Autodesk Inventor part; units mm, degrees
ref_plane "YZ Plane" through (0, 0, 0) normal (1, 0, 0) x (0, 1, 0)
ref_plane "XZ Plane" through (0, 0, 0) normal (0, 1, 0) x (-1, 0, 0)
ref_plane "XY Plane" through (0, 0, 0) normal (0, 0, 1) x (1, 0, 0)
sketch "Sketch2" plane through (0, 0, 0) normal (1, 0, 0) x (0, 1, 0)
  line L0 (0, 0) -> (1, 0)
  line L1 (1, 0) -> (1, 1)
  line L2 (1, 1) -> (2.25, 1)
  line L3 (2.25, 1) -> (2.25, 3)
  line L4 (2.25, 3) -> (3, 3)
  line L5 (3, 3) -> (3, 13)
  line L6 (3, 13) -> (0, 13)
  line L7 (0, 13) -> (0, 0)
  arc A0 (1, 0) -> (2.25, 1) centre (0.8455, 1.4743) ccw
  dimension "d3" = 1
  dimension "d4" = 1
  dimension "d5" = 1.25
  dimension "d6" = 2
  dimension "d7" = 0.75
  dimension "d8" = 10
  dimension "d9" = 3
revolve "Revolution1" add sketch "Sketch2" angle 360 about axis through (0, 0, 13) along (0, 0, -1)
thread "Thread1"
sketch "Sketch3" plane through (0, 0, 13) normal (0, 0, 1) x (1, 0, 0)
  line L0 (2.8868, 5) -> (5.7735, 0)
  line L1 (5.7735, 0) -> (2.8868, -5)
  line L2 (2.8868, -5) -> (-2.8868, -5)
  line L3 (-2.8868, -5) -> (-5.7735, 0)
  line L4 (-5.7735, 0) -> (-2.8868, 5)
  line L5 (-2.8868, 5) -> (2.8868, 5)
  point P0 (0, 0)
  point P1 (0, 0)
  dimension "d13" = 10
extrude "Extrusion2" add sketch "Sketch3" along normal blind 3.5
chamfer "Chamfer1" distance 0.5 angle 45 6 edges at (0, 5, 16.5) (4.3301, 2.5, 16.5) (4.3301, -2.5, 16.5) (0, -5, 16.5) (-4.3301, -2.5, 16.5) (-4.3301, 2.5, 16.5)
sketch "Sketch4" plane through (0, 0, 16.5) normal (0, 0, 1) x (1, 0, 0)
  circle A0 centre (0, 0) radius 2
  dimension "d19" = 4
extrude "Extrusion3" add sketch "Sketch4" along normal blind 8
properties part number "Termocupla" material "Steel"
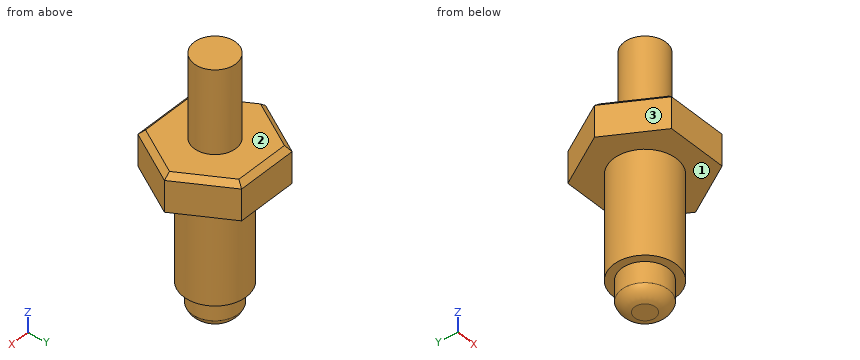
The model under review builds one solid part; all positions refer to its coordinate system, in mm. Face numbers are marked on the shaded views. A direction names the side the tool comes from. Round coordinates to 2 decimals unless told otherwise and drop trailing zeros. Loops run counter-clockwise (first coordinate to the right, second up) from the corner with the lowest first, then second, coordinate; pieces in that order, holes last. Notation, with made-up numbers: M 54,-26.5 L 110,-26.5 A38 cw 110,12.5 Z; hole C 37.25,44.25 d9. An arc over 180 degrees is marked long. Write item = value, one per line.
Item 1: Take a section at D-D on z = 10.5. Write out the cut boundary in (x, y).
Return value:
outline = C 0,0 d6
Item 2: Insertion check: P1, Ø3, axis at x = 1.5, z = 20.5, coming from the -Y side; P2, Ø2, axis at x = -1, y = -3.5, coming from the -Z side; P3, Ø2, axis at x = 1.5, z = 3.5, coming from the +Y side. Each pin has a flat end and moves straight along its axis. Give the tip position at first contact, or say it passes through.
Return value:
P1 = -2
P2 = 3
P3 = 2.96
Item 3: For line 1 (Z direction, x = 2.5, y = 1.75); line 2 (Z direction, x = 1.75, y = -2); line 3 (Y direction, x = 2, z = 12.25), list the stretches that pass through material, from the lowest coordinate up. Write a range as [from, to].
Return value:
line_1 = [13, 16.5]
line_2 = [3, 16.5]
line_3 = [-2.24, 2.24]
Item 4: Take a section at B-B on y = 4. Write out the cut boundary in (x, z).
Return value:
outline = M -3.46,13 L 3.46,13 L 3.46,16 L 2.89,16.5 L -2.89,16.5 L -3.46,16 Z
Item 5: Machinability: for the marked faces 1, 2 and 3, which of the approach directions +Z, -Z, +X, -X, +Y, -Y give a long, thin tool a straight path to every point of the face, cutting with its end or side? Answer none if there is none.
Return value:
face_1 = -Z
face_2 = +Z
face_3 = +Z, -Z, -X, -Y
Item 6: Take a section at C-C on z = 20.5. Write out the cut boundary in (x, y), then the cut area to 3 significant figures.
Return value:
outline = C 0,0 d4
area = 12.6 mm2
Item 7: Take a section at A-A on z = 13.75. Write out the cut boundary in (x, y).
Return value:
outline = M -5.77,0 L -2.89,-5 L 2.89,-5 L 5.77,0 L 2.89,5 L -2.89,5 Z
